Work out the finished part from the listing and answer in its coordinate system (mm). A direction names the side the tool comes from. Coordinates: 2 decimals unless noted, no trailing zeros. Order: outer loops, then holes, each group sorted by start corner. A loop starts at its lowest first (then second) coordinate and runs counter-clockwise, first axis right, second up. Notation, with made-up numbers: (65.25, 76) -> (83.25, 76) arc R19 ccw to (83.25, 103) -> close; hole circle Ø11 at (34, 35). An arc over 180 degrees is marked (long way). Use one line per item in the form item = value.
from build123d import *

# Parameters (mm, degrees)
F0_R      = 25
F0_R_2    = 3
F0_R_3    = 12.5
F1_DEPTH  = 20
F2_R      = 25
F2_R_2    = 12.5
F3_DEPTH  = 10
F4_SIZE2  = 10
F4_SIZE   = 5
F5_R      = 4
F6_DEPTH  = 26.0000001
F8_R      = 7
F9_DEPTH  = 5
F10_DEPTH = 20


with BuildPart() as f1:
    # F0 (on Top) → F1 (new body)
    with BuildSketch(Plane.XY):
        Circle(F0_R)
        with Locations((-15.5884572681, -9)):
            Circle(F0_R_2, mode=Mode.SUBTRACT)
        with Locations((0, -18)):
            Circle(F0_R_2, mode=Mode.SUBTRACT)
        with Locations((15.5884572681, -9)):
            Circle(F0_R_2, mode=Mode.SUBTRACT)
        with Locations((-15.5884572681, 9)):
            Circle(F0_R_2, mode=Mode.SUBTRACT)
        Circle(F0_R_3, mode=Mode.SUBTRACT)
        with Locations((15.5884572681, 9)):
            Circle(F0_R_2, mode=Mode.SUBTRACT)
        with Locations((0, 18)):
            Circle(F0_R_2, mode=Mode.SUBTRACT)
        with Locations((0, -18)):
            Circle(F0_R_2)
        with Locations((-15.5884572681, -9)):
            Circle(F0_R_2)
        with Locations((15.5884572681, -9)):
            Circle(F0_R_2)
        with Locations((15.5884572681, 9)):
            Circle(F0_R_2)
        with Locations((0, 18)):
            Circle(F0_R_2)
        with Locations((-15.5884572681, 9)):
            Circle(F0_R_2)
    extrude(amount=F1_DEPTH)

    # F2 (on face) → F3 (join)
    with BuildSketch(Plane.XY.offset(20)):
        Circle(F2_R)
        Circle(F2_R_2, mode=Mode.SUBTRACT)
    extrude(amount=F3_DEPTH)

    # F4
    f4_edges = [f1.edges().sort_by_distance(p)[0] for p in [
        (-25, 0, 30),
    ]]
    f4_side = f1.faces().sort_by_distance((-24.292893, 0, 30))[0]
    chamfer(f4_edges, length=F4_SIZE, length2=F4_SIZE2, reference=f4_side)

    # F5 (on Right) → F6 (cut, up to face)
    with BuildSketch(Plane.YZ):
        with Locations((0, 12)):
            Circle(F5_R)
    extrude(amount=-F6_DEPTH, mode=Mode.SUBTRACT)

    # F8 (on offset) → F9 (cut)
    with BuildSketch(Plane.YZ.offset(-25)):
        with Locations((0, 12)):
            Circle(F8_R)
    extrude(amount=F9_DEPTH, mode=Mode.SUBTRACT)

    # F0 (on Top) → F10 (cut)
    with BuildSketch(Plane.XY):
        with Locations((0, -18)):
            Circle(F0_R_2)
        with Locations((15.5884572681, -9)):
            Circle(F0_R_2)
        with Locations((15.5884572681, 9)):
            Circle(F0_R_2)
        with Locations((0, 18)):
            Circle(F0_R_2)
        with Locations((-15.5884572681, 9)):
            Circle(F0_R_2)
        with Locations((-15.5884572681, -9)):
            Circle(F0_R_2)
    extrude(amount=F10_DEPTH, mode=Mode.SUBTRACT)


solid = f1.part
(1) Which of the six approach directions +Z, -Z, +X, -X, +Y, -Y give full straight-line access (tool end or side, diameter ignored) to faces 4 (the flat face through (-11.5, 5.9, 0)), 5 (the flat face through (0, 18, 20)), 6 (the cylindrical face through (-16, -4, 12))?
Data:
face_4 = -Z, +X, -X, +Y, -Y
face_5 = -Z
face_6 = -X
(2) Each of these flat-tipped pins is pushed along its axis until it touches: P1, Ø6, axis at y = -1, z = 25.5, coming from the +X side; P2, Ø20, axis at x = 0, y = 0, coming from the +Z side; P3, Ø6, axis at y = 10.5, z = 14, coming from the +X side; P4, Ø4, axis at y = 14, z = 13.5, coming from the +X side. Where does it stop, or does it pass through?
Data:
P1 = 23.73
P2 = through
P3 = 23.85
P4 = 21.93
(3) Section B-B on y = 0 is taken. Write down the section's boundary in (x, z).
Data:
outline = (-25, 0) -> (-12.5, 0) -> (-12.5, 8) -> (-20, 8) -> (-20, 5) -> (-25, 5) -> close; (-25, 19) -> (-20, 19) -> (-20, 16) -> (-12.5, 16) -> (-12.5, 30) -> (-20, 30) -> (-25, 20) -> close; (12.5, 0) -> (25, 0) -> (25, 20) -> (20, 30) -> (12.5, 30) -> close
(4) The mould has two halves that part along Y. Classify faces 1 (the flat face through (-9, -9, 30)), 2 (the cylindrical face through (23.846, 7.509, 9.86)), 3 (the cylindrical face through (-22.535, -5.555, 7.741)): released by +Y, released by -Y, zero draft, split by the parting line, or undercut.
Data:
face_1 = zero draft
face_2 = split by the parting line
face_3 = undercut
(5) Section D-D on z = 21 is taken. Write down the section's boundary in (x, y), plus the area to 3 significant figures.
Data:
outline = circle Ø49 at (0, 0); hole circle Ø25 at (0, 0)
area = 1,390 mm²
(6) Section A-A on x = 0 is taken. Write down the section's boundary in (y, z), plus the area to 3 significant figures.
Data:
outline = (-25, 0) -> (-21, 0) -> (-21, 20) -> (-15, 20) -> (-15, 0) -> (-12.5, 0) -> (-12.5, 30) -> (-20, 30) -> (-25, 20) -> close; (12.5, 0) -> (15, 0) -> (15, 20) -> (21, 20) -> (21, 0) -> (25, 0) -> (25, 20) -> (20, 30) -> (12.5, 30) -> close
area = 460 mm²
(7) Section C-C on z = 12 is taken. Write down the section's boundary in (x, y).
Data:
outline = (-24, -7) arc R25 ccw (long way) to (-24, 7) -> (-20, 7) -> (-20, 4) -> (-11.84, 4) arc R12.5 cw (long way) to (-11.84, -4) -> (-20, -4) -> (-20, -7) -> close; hole circle Ø6 at (-15.59, -9); hole circle Ø6 at (-15.59, 9); hole circle Ø6 at (0, -18); hole circle Ø6 at (0, 18); hole circle Ø6 at (15.59, -9); hole circle Ø6 at (15.59, 9)
(8) Straight lines are drawn through the part: line 1 along Y through (x, z) = (0, 9); line 2 along Y through (x, z) = (2.5, 16); line 3 along X through (y, z) = (-5, 16.5). For each, find the intervals that lie inside material, in ascending order.
Data:
line_1 = -25 to -21, -15 to -12.5, 12.5 to 15, 21 to 25
line_2 = -24.87 to -19.66, -16.34 to -12.25, 12.25 to 16.34, 19.66 to 24.87
line_3 = -20 to -11.46, 11.46 to 24.49
